Can you work these out from the model? Positions are in its coordinate system, mm. Face numbers are marked on the shaded views. Round coordinates to 2 decimals unless told otherwise and drop trailing zeros. Write each loop counter-clockwise with the first axis right and the second up, starting at its lowest first coordinate (ties: lowest second). Pieces come first, ordered by that corner, then holes. Notation, with made-up numbers: M 44,-36 L 61,-36 A28 cw 61,-5 Z; hole C 31,86.25 d1. An arc over 180 degrees is marked long. Answer in a Markdown table with one row per item. Add a question column.
(1) If we mould it in two halves opening along X, with no side actions, what happens to the marked faces 1 and 2? For each: released by +X, released by -X, zero draft, split by the parting line, or undercut.
(2) Suppose I cut it at C-C, the plane y = 0.75. Write out the boundary of the cut face in (x, z).
(3) Suppose I cut it at B-B, the plane x = 7. Write out the boundary of the cut face in (y, z).
(4) If I drill on probe 1 along X at (y, z) = (0.45, -7); probe 2 along X at (y, z) = (0.15, 7), over which ranges is the centre line in solid material (lowest first)?
(5) Suppose I cut it at D-D, the plane z = 4. Write out the boundary of the cut face in (x, y).
(6) Suppose I cut it at A-A, the plane z = 7. Write out the boundary of the cut face in (x, y), then the cut area to 3 significant figures.
(7) I'm going to push flat-ended pins straight in: pin 1 (3.5 mm diameter, centred on x = -7, z = 7, fed in from -Y); pin 2 (5 mm diameter, centred on x = -1.5, z = 3, fed in from -Y). Where does each tip first touch, or does it pass through?
from build123d import *

# Parameters (mm, degrees)
SKETCH_1_W              = 20
SKETCH_1_H              = 20
EXTRUDE_1_DEPTH         = 1.5
SKETCH_2_W              = 10.1
SKETCH_2_H              = 17.5
CUT_EXTRUDE_1_DEPTH     = 0.25
HOLE_WIZARD_3_2_3_2_1_D = 3.2
HOLE_WIZARD_3_2_3_2_2_D = 3.2


with BuildPart() as part:
    # 草图1 → 凸台-拉伸1 (new body)
    with BuildSketch(Plane.XZ):
        Rectangle(SKETCH_1_W, SKETCH_1_H)
    extrude(amount=-EXTRUDE_1_DEPTH)

    # 草图2 → 切除-拉伸1 (cut)
    with BuildSketch(Plane.XZ):
        with Locations((0, 1.25)):
            Rectangle(SKETCH_2_W, SKETCH_2_H)
    extrude(amount=-CUT_EXTRUDE_1_DEPTH, mode=Mode.SUBTRACT)

    # Ø3.2 (3.2) 直径孔1 (through all)
    with Locations(Plane(origin=(0, 1.5, 0), x_dir=(1, 0, 0), z_dir=(0, 1, 0))):
        with Locations((-7, -7), (7, 7)):
            Hole(HOLE_WIZARD_3_2_3_2_1_D / 2)

    # Ø3.2 (3.2) 直径孔2 (through all)
    with Locations(Plane(origin=(0, 0, 0), x_dir=(-1, 0, 0), z_dir=(0, -1, 0))):
        with Locations((-7, -7), (7, 7)):
            Hole(HOLE_WIZARD_3_2_3_2_2_D / 2)


solid = part.part
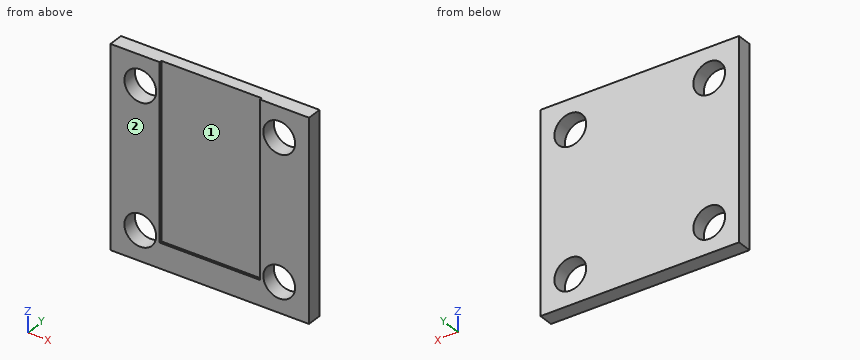
Calculated:
| question | item | result |
|---|---|---|
| 1 | face 1 | undercut |
| 1 | face 2 | zero draft |
| 2 | outline | M -10,-10 L 10,-10 L 10,10 L -10,10 Z; hole C -7,-7 d3.2; hole C -7,7 d3.2; hole C 7,-7 d3.2; hole C 7,7 d3.2 |
| 3 | outline | M 0,-10 L 1.5,-10 L 1.5,-8.6 L 0,-8.6 Z; M 0,-5.4 L 1.5,-5.4 L 1.5,5.4 L 0,5.4 Z; M 0,8.6 L 1.5,8.6 L 1.5,10 L 0,10 Z |
| 4 | probe 1 | -10 to -8.6, -5.4 to 5.4, 8.6 to 10 |
| 4 | probe 2 | -10 to -8.6, -5.4 to -5.05, 5.05 to 5.4, 8.6 to 10 |
| 5 | outline | M -10,0 L -5.05,0 L -5.05,0.25 L 5.05,0.25 L 5.05,0 L 10,0 L 10,1.5 L -10,1.5 Z |
| 6 | outline | M -10,0 L -8.6,0 L -8.6,1.5 L -10,1.5 Z; M -5.4,0 L -5.05,0 L -5.05,0.25 L 5.05,0.25 L 5.05,0 L 5.4,0 L 5.4,1.5 L -5.4,1.5 Z; M 8.6,0 L 10,0 L 10,1.5 L 8.6,1.5 Z |
| 6 | area | 17.9 mm² |
| 7 | pin 1 | y = 0 |
| 7 | pin 2 | y = 0.25 |
